Input: part model. Units: mm. Frame: model coordinates. A direction names the side the tool comes from. Give positions to 0.01 mm unless a question says otherwise; leave off trailing zeros. Loops run counter-clockwise (first coordinate to the right, second up) from the corner with the lowest first, then second, coordinate; pieces in that order, holes last. Notation, with made-up numbers: M 12.5,87 L 20.5,87 A20 cw 20.5,118 Z; hole C 15.5,58.5 d3. An arc over 180 degrees is marked long. One line per item, written item: value. Start each with the question number.
(1) Ray query, line 1 along Z through (x, y) = (0, -1.65); line 2 along Z through (x, y) = (0, -7); line 3 along Y through (x, z) = (38, 16). Return the intervals inside material, ascending. Write a range as from..to.
(2) Section C-C on y = -5. Output: boundary loops of the cut face in (x, z).
(3) Section D-D on z = -11. Output: boundary loops of the cut face in (x, y).
(4) Section B-B on z = 0. Output: boundary loops of the cut face in (x, y).
(5) Pull-direction query (Z, two-part tool) for faces 4 (the flat face through (-0.3, 0, -5.2)), 5 (the cylindrical face through (-23.846, -4.93, 7.509)), 6 (the cylindrical face through (1.08, -1.48, -4.88)); classes: released by +Z, released by -Z, zero draft, split by the parting line, or undercut.
(6) Access query for faces 1 (the cylindrical face through (-10.3, -11.48, -46.37)), 2 (the cylindrical face through (-14.985, -8.07, 0.66)), 3 (the flat face through (-20, -10, -20)). Directions: +Z, -Z, +X, -X, +Y, -Y. A direction counts if a zero-diameter tool reaches every point of the face in a straight line with its end or side. Return the directions, or none.
(7) Pin query (flat end, axial travel): P1, Ø2, axis at x = -3, y = -8.5, coming from the -Z side; P2, Ø3, axis at y = -11, z = -9.5, coming from the -X side; P3, Ø10, axis at x = -19.5, z = 35, coming from the +Y side. Return the tip coordinate at first contact, or that it passes through.
(8) Section A-A on x = 0. Output: boundary loops of the cut face in (y, z).
```python
from build123d import *

# Parameters (mm, degrees)
F0_R     = 47.5
F1_DEPTH = 13
F2_R     = 15
F3_DEPTH = 10
F4_R     = 58.550263
F4_R_2   = 25
F5_DEPTH = 10
F6_R     = 5
F7_DEPTH = 25


with BuildPart() as f1:
    # F0 (on Front) → F1 (new body)
    with BuildSketch(Plane.XZ):
        Circle(F0_R)
    extrude(amount=F1_DEPTH)

    # F2 (on face) → F3 (cut)
    with BuildSketch(Plane.XZ.offset(13)):
        Circle(F2_R)
    extrude(amount=-F3_DEPTH, mode=Mode.SUBTRACT)

    # F4 (on face) → F5 (cut)
    with BuildSketch(Plane(origin=(0, 0, 0), x_dir=(-1, 0, 0), z_dir=(0, 1, 0))):
        with Locations((0, -4.284165)):
            Circle(F4_R)
        Circle(F4_R_2, mode=Mode.SUBTRACT)
    extrude(amount=-F5_DEPTH, mode=Mode.SUBTRACT)

    # F6 (on face) → F7 (cut)
    with BuildSketch(Plane(origin=(0, 0, 0), x_dir=(-1, 0, 0), z_dir=(0, 1, 0))):
        Circle(F6_R)
    extrude(amount=-F7_DEPTH, mode=Mode.SUBTRACT)


solid = f1.part
```
Output values:
1. line 1: z = -25..-5, 5..25
1. line 2: z = -25..-15, 15..25
1. line 3: y = -13..-10
2. outline: C 0,0 d50; hole C 0,0 d30
3. outline: M -46.21,-13 L -10.2,-13 L -10.2,-3 L 10.2,-3 L 10.2,-13 L 46.21,-13 L 46.21,-10 L 22.45,-10 L 22.45,0 L -22.45,0 L -22.45,-10 L -46.21,-10 Z
4. outline: M -47.5,-13 L -15,-13 L -15,-3 L -5,-3 L -5,0 L -25,0 L -25,-10 L -47.5,-10 Z; M 5,-3 L 15,-3 L 15,-13 L 47.5,-13 L 47.5,-10 L 25,-10 L 25,0 L 5,0 Z
5. face 4: zero draft
5. face 5: split by the parting line
5. face 6: undercut
6. face 1: +Y, -Y
6. face 2: -Y
6. face 3: +Y
7. P1: stops at z = -24.92
7. P2: stops at x = -46.82
7. P3: stops at y = -10
8. outline: M -13,-47.5 L -10,-47.5 L -10,-25 L 0,-25 L 0,-5 L -3,-5 L -3,-15 L -13,-15 Z; M -13,15 L -3,15 L -3,5 L 0,5 L 0,25 L -10,25 L -10,47.5 L -13,47.5 Z
